```python
from build123d import *

# Parameters (mm, degrees)
SKETCH1_R             = 1.35
BOSS_EXTRUDE2_DEPTH   = 13
BOSS_EXTRUDE2_2_DEPTH = 13
SKETCH4_R             = 1.35
BOSS_EXTRUDE5_DEPTH   = 3


with BuildPart() as part:
    # Sketch1 → Boss-Extrude2 (new body)
    with BuildSketch(Plane(origin=(0, 0, 0), x_dir=(1, 0, 0), z_dir=(0, 1, 0))):
        Polygon((-11.255, 23.58), (-29.745, 23.58), (-29.745, 16.589209278), (-22.7039371, 16.589209278), (-22.7039371, -16.42), (-29.745, -16.42), (-29.745, -23.58), (-11.255, -23.58), (-11.255, -20.58), (-17.255, -20.58), (-17.255, 20.58), (-11.255, 20.58), align=None)
        with Locations(Location((-26.22446855, 20.084604639, 0), (0, 0, 90))):
            Circle(SKETCH1_R, mode=Mode.SUBTRACT)
        with Locations(Location((-26.22446855, -19.915395361, 0), (0, 0, 90))):
            Circle(SKETCH1_R, mode=Mode.SUBTRACT)
    extrude(amount=BOSS_EXTRUDE2_DEPTH)



with BuildPart() as body_2:
    # Sketch1 → Boss-Extrude2 2 (new body)
    with BuildSketch(Plane(origin=(0, 0, 0), x_dir=(1, 0, 0), z_dir=(0, 1, 0))):
        Polygon((14.255, 23.58), (14.255, 20.58), (17.255, 20.58), (17.255, -20.58), (14.255, -20.58), (14.255, -23.58), (27.2960629, -23.58), (27.2960629, -16.42), (20.255, -16.42), (20.255, 16.589209278), (27.2960629, 16.589209278), (27.2960629, 23.58), align=None)
        with Locations(Location((23.77553145, 20.084604639, 0), (0, 0, 90))):
            Circle(SKETCH1_R, mode=Mode.SUBTRACT)
        with Locations(Location((23.77553145, -19.915395361, 0), (0, 0, 90))):
            Circle(SKETCH1_R, mode=Mode.SUBTRACT)
    extrude(amount=BOSS_EXTRUDE2_2_DEPTH)


with BuildPart() as part_1:
    add(part.part)

    add(body_2.part)  # Boss-Extrude5 merges body 2
    # Sketch4 → Boss-Extrude5 (add)
    # profile 1 of 4: a face of its own
    with BuildSketch(Plane(origin=(0, 13, 0), x_dir=(1, 0, 0), z_dir=(0, 1, 0))):
        Polygon((-29.745, -23.58), (-11.255, -23.58), (-11.255, -20.58), (-17.255, -20.58), (-17.255, 20.58), (-11.255, 20.58), (-11.255, 23.58), (-29.745, 23.58), (-29.745, 16.589209278), (-22.7039371, 16.589209278), (-22.7039371, -16.42), (-29.745, -16.42), align=None)
        with Locations(Location((-26.22446855, -19.915395361, 0), (0, 0, 90))):
            Circle(SKETCH4_R, mode=Mode.SUBTRACT)
        with Locations(Location((-26.22446855, 20.084604639, 0), (0, 0, 90))):
            Circle(SKETCH4_R, mode=Mode.SUBTRACT)
    # profile 2 of 4: a face of its own
    with BuildSketch(Plane(origin=(0, 13, 0), x_dir=(1, 0, 0), z_dir=(0, 1, 0))):
        Polygon((27.2960629, 23.58), (-11.255, 23.58), (-11.255, 20.58), (-17.255, 20.58), (-17.255, -20.58), (-11.255, -20.58), (-11.255, -23.58), (27.2960629, -23.58), (27.2960629, -16.42), (20.255, -16.42), (20.255, 16.589209278), (27.2960629, 16.589209278), align=None)
    # profile 3 of 4: a face of its own
    with BuildSketch(Plane(origin=(0, 13, 0), x_dir=(1, 0, 0), z_dir=(0, 1, 0))):
        with Locations(Location((-26.22446855, 20.084604639, 0), (0, 0, 90))):
            Circle(SKETCH4_R)
    # profile 4 of 4: a face of its own
    with BuildSketch(Plane(origin=(0, 13, 0), x_dir=(1, 0, 0), z_dir=(0, 1, 0))):
        with Locations(Location((-26.22446855, -19.915395361, 0), (0, 0, 90))):
            Circle(SKETCH4_R)
    extrude(amount=BOSS_EXTRUDE5_DEPTH)


solid = part_1.part
```
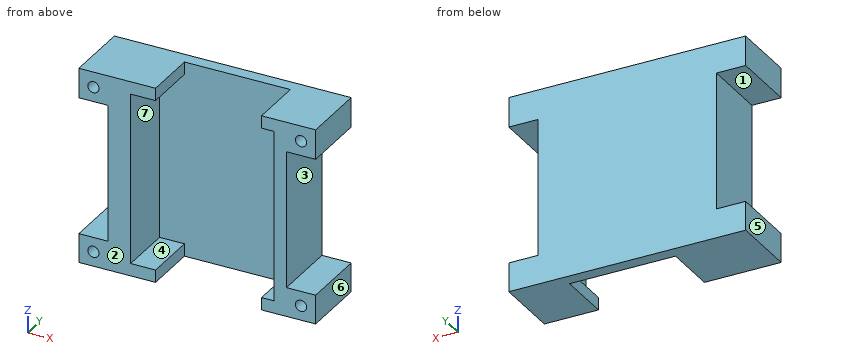
Can you work these out from the model? Positions are in its coordinate system, mm. Face numbers are marked on the shaded views. A direction names the side the tool comes from. Give positions to 0.01 mm unless a question says otherwise; leave off trailing zeros. Loops run counter-clockwise (first coordinate to the right, second up) from the corner with the lowest first, then second, coordinate; pieces in that order, holes last. Notation, with made-up numbers: M 29,-22.75 L 50,-22.75 A22 cw 50,-5.75 Z; hole C 86.5,-3 d3. An arc over 180 degrees is marked long. One line per item, written item: value.
(1) Suppose I cut it at A-A on y = 2. List the corners of the cut face in (x, z) for me (3 decimals), plus the area to 3 significant figures.
Returned:
outline: M -29.745,-23.58 L -11.255,-23.58 L -11.255,-20.58 L -17.255,-20.58 L -17.255,20.58 L -11.255,20.58 L -11.255,23.58 L -29.745,23.58 L -29.745,16.42 L -22.704,16.42 L -22.704,-16.589 L -29.745,-16.589 Z; M 14.255,-23.58 L 27.296,-23.58 L 27.296,-16.589 L 20.255,-16.589 L 20.255,16.42 L 27.296,16.42 L 27.296,23.58 L 14.255,23.58 L 14.255,20.58 L 17.255,20.58 L 17.255,-20.58 L 14.255,-20.58 Z; hole C -26.224,-20.085 d2.7; hole C -26.224,19.915 d2.7; hole C 23.776,-20.085 d2.7; hole C 23.776,19.915 d2.7
area: 629 mm^2
(2) We'd pull the mould along X, two halves only. Please class the marked faces 5, 6 and 7: released by +X, released by -X, zero draft, split by the parting line, or undercut.
Returned:
face 5: released by -X
face 6: released by +X
face 7: undercut
(3) I need wall thicknesses on line 1 (X direction, y = 11, z = 12) (3 decimals); line 2 (Z direction, x = -11.5, y = 4.25); line 3 (X direction, y = 9.5, z = -19.5) (3 decimals). Which ranges of each line are inside material? Lowest first, please.
Returned:
line 1: -22.704 to -17.255, 17.255 to 20.255
line 2: -23.58 to -20.58, 20.58 to 23.58
line 3: -29.745 to -27.441, -25.008 to -17.255, 17.255 to 22.559, 24.992 to 27.296
(4) Suppose I cut it at C-C on y = 14.5. List the corners of the cut face in (x, z) for me (3 decimals), plus the area to 3 significant figures.
Returned:
outline: M -29.745,-23.58 L 27.296,-23.58 L 27.296,-16.589 L 20.255,-16.589 L 20.255,16.42 L 27.296,16.42 L 27.296,23.58 L -29.745,23.58 L -29.745,16.42 L -22.704,16.42 L -22.704,-16.589 L -29.745,-16.589 Z
area: 2,230 mm^2
(5) Will this pin go through, and if not, where does the flat tip stop? pin 1 (12 mm diameter, centred on x = -7.5, z = 11.5, fed in from -Y).
Returned:
pin 1: y = 13
(6) Which directions (+Z, -Z, +X, -X, +Y, -Y) give clear straight access to the entire face, cutting with the end or side of a thin tool? Please do the marked faces 1, 2, 3 and 4.
Returned:
face 1: -X, +Y, -Y
face 2: +Z, -Z, +X, -X, -Y
face 3: +X, +Y, -Y
face 4: -Y
(7) Suppose I cut it at B-B on z = 11. List the corners of the cut face in (x, y) for me (3 decimals), plus the area to 3 significant figures.
Returned:
outline: M -22.704,0 L -17.255,0 L -17.255,13 L 17.255,13 L 17.255,0 L 20.255,0 L 20.255,16 L -22.704,16 Z
area: 239 mm^2
(8) Suppose I cut it at D-D on x = -7.5. List the corners of the cut face in (y, z) for me, plus the area to 3 significant figures.
Returned:
outline: M 13,-23.58 L 16,-23.58 L 16,23.58 L 13,23.58 Z
area: 141 mm^2
